```python
from build123d import *

# Parameters (mm, degrees)
F1_DEPTH = 770


with BuildPart() as f1:
    # F0 (on Front) → F1 (new body)
    with BuildSketch(Plane.XZ):
        Polygon((20, 5), (20, 20), (5, 20), (5, 15), (10, 15), (5, 10), (-5, 10), (-10, 15), (-5, 15), (-5, 20), (-20, 20), (-20, 5), (-15, 5), (-15, 10), (-10, 5), (-10, -5), (-15, -10), (-15, -5), (-20, -5), (-20, -20), (-5, -20), (-5, -15), (-10, -15), (-5, -10), (5, -10), (10, -15), (5, -15), (5, -20), (20, -20), (20, -5), (15, -5), (15, -10), (10, -5), (10, 5), (15, 10), (15, 5), align=None)
        Polygon((-5, 0), (-5, 5), (0, 5), (5, 5), (5, 0), (5, -5), (0, -5), (-5, -5), align=None, mode=Mode.SUBTRACT)
    extrude(amount=F1_DEPTH)


solid = f1.part
```
Read the model definition and answer for the solid it produces. Units are mm, in the model's axes. Round coordinates to 2 decimals unless told otherwise and drop trailing zeros. One line per item, written item: value.
Q1. Straight lines are drawn through the part: line 1 (Z direction, x = -15.5, y = -43); line 2 (Z direction, x = -1.5, y = -123). For each, find the intervals that lie inside material, in ascending order. Write a range as [from, to].
Data:
line 1: [-20, -5], [5, 20]
line 2: [-10, -5], [5, 10]
Q2. Flat-ended cylindrical pins translate along their axes: pin 1 Ø5 at (x, y) = (-0.5, -427.5) entering from +Z; pin 2 Ø1.5 at (x, y) = (-2.5, -198) entering from -Z; pin 3 Ø5 at (y, z) = (-403.5, 0.5) entering from -X. Find the tip coordinate at first contact, or state that the pin passes through.
Data:
pin 1: z = 10
pin 2: z = -10
pin 3: x = -10
Q3. For a pull along X with two mould halves and no side action, classify faces 1 (the flat face through (9, 0, 0)), 2 (the flat face through (-20, -380, 13)), 3 (the flat face through (20, -380, 12)) as +X half, -X half, draft (parallel to the pull), parting line (faces both ways), or undercut.
Data:
face 1: draft
face 2: -X half
face 3: +X half
